Input: part model. Units: mm. Frame: model coordinates. A direction names the side the tool comes from. Coordinates: 2 decimals unless noted, no trailing zeros. Order: outer loops, then holes, each group sorted by start corner. A loop starts at its lowest first (then second) coordinate and runs counter-clockwise, first axis right, second up. Notation, with made-up numbers: (88.5, 41.25) -> (120.5, 41.25) arc R24 ccw to (120.5, 65.25) -> close; hole circle Ø1 at (-30, 18). An arc over 180 degrees is marked (long way). Use one line per item in the form item = value. Start each with the question number.
1) Draft query along Z for faces 4 (the cylindrical face through (16.6, 3.52, 19.93)), 5 (the cylindrical face through (0.96, 5.74, 9.23)), 6 (the cylindrical face through (-18.63, 0.6, 0.26)). Return one class per face: pulls with the +Z half, pulls with the -Z half, needs draft (parallel to the pull), parting line crosses it, or undercut.
2) Access query for faces 1 (the flat face through (0, 3, -15)), 2 (the cylindrical face through (0.96, 5.74, -16.77)), 3 (the flat face through (-17, 18, 0.5)). Directions: +Z, -Z, +X, -X, +Y, -Y. A direction counts if a zero-diameter tool reaches every point of the face in a straight line with its end or side. Return the directions, or none.
3) Section query D-D on z = 6. Output: boundary loops of the cut face in (x, y).
4) Section query B-B on z = 13. Output: boundary loops of the cut face in (x, y).
5) Section query A-A on y = 23.5. Output: boundary loops of the cut face in (x, z), then the cut area to 3 significant figures.
6) Pin query (flat end, axial travel): pin 1 (18 mm diameter, centred on x = -4, z = 3, fed in from +Y); pin 2 (12 mm diameter, centred on x = 9, y = 13, fed in from +Z); pin 3 (1 mm diameter, centred on x = 9, z = -6.5, fed in from +Y). Return the tip coordinate at first contact, or that it passes through.
7) Ray query, line 1 along X through (y, z) = (6.2, 13); line 2 along Z through (x, y) = (-1, 6.55); line 3 along X through (y, z) = (5.25, -13). Return the intervals inside material, ascending.
8) Section query C-C on x = -1. Count the separate pieces of the cut face and the enclosed holes in it, then the cut area to 3 significant figures.
Autodesk Inventor part; units mm, degrees
ref_plane "YZ Plane" through (0, 0, 0) normal (1, 0, 0) x (0, 1, 0)
ref_plane "XZ Plane" through (0, 0, 0) normal (0, 1, 0) x (-1, 0, 0)
ref_plane "XY Plane" through (0, 0, 0) normal (0, 0, 1) x (1, 0, 0)
sketch "Sketch1" plane through (0, 0, 0) normal (0, 1, 0) x (-1, 0, 0)
  line L0 (19.2, 20.5) -> (-17.2, 20.5)
  line L1 (-17.2, 20.5) -> (-17.2, -20.5)
  line L2 (-17.2, -20.5) -> (19.2, -20.5)
  line L3 (19.2, -20.5) -> (19.2, 20.5)
  point P0 (0, 0)
  dimension "d0" = 36.4
  dimension "d1" = 41
extrude "Extrusion1" add sketch "Sketch1" along normal blind 5
sketch "Sketch2" plane through (0, 5, 0) normal (0, 1, 0) x (1, 0, 0)
  line L0 (-19.2, -20.5) -> (17.2, -20.5)
  line L1 (-19.2, -20.5) -> (-14.2, -20.5)
  line L2 (-14.2, -20.5) -> (-14.2, -0.5)
  line L3 (-14.2, -0.5) -> (-19.2, -0.5)
  line L4 (-19.2, -0.5) -> (-19.2, -20.5)
  line L5 (17.2, 20.5) -> (-19.2, 20.5)
  line L6 (17.2, 20.5) -> (12.2, 20.5)
  line L7 (12.2, 20.5) -> (12.2, 0.5)
  line L8 (12.2, 0.5) -> (17.2, 0.5)
  line L9 (17.2, 0.5) -> (17.2, 20.5)
  point P0 (0, 0)
  dimension "d4" = 5
  dimension "d5" = 20
  dimension "d6" = 5
  dimension "d7" = 20
extrude "Extrusion2" add sketch "Sketch2" along normal blind 25.4
sketch "Sketch3" plane through (0, 5, 0) normal (0, 1, 0) x (1, 0, 0)
  circle A0 centre (-1, -13) radius 4.25
  circle A1 centre (-1, 13) radius 4.25
  line L0 (-14.2, -20.5) -> (-14.2, -0.5)
  line L1 (12.2, 20.5) -> (12.2, 0.5)
  point P0 (0, 0)
  dimension "d10" = 8.5
  dimension "d11" = 8.5
  dimension "d24" = 13.2
  dimension "d25" = 13.2
extrude "Extrusion3" add sketch "Sketch3" along normal blind 3
sketch "Sketch4" plane through (-1, 8, 13) normal (0, 1, 0) x (1, 0, 0)
  circle A0 centre (0, 0) radius 4.25
  circle A1 centre (0, 0) radius 2
  circle A2 centre (0, 26) radius 4.25
  circle A3 centre (0, 26) radius 2
  point P0 (1, 13)
  dimension "d14" = 4
  dimension "d15" = 4
extrude "Extrusion4" cut sketch "Sketch4" against normal blind 10 contours A1 | A3
fillet "Fillet1" radius 2 8 edges at (17.2, 0, 0) (-1, 0, 20.5) (-19.2, 0, 0) (-1, 0, -20.5) (-19.2, 15.2, 20.5) (17.2, 15.2, -20.5) (-19.2, 2.5, -20.5) (17.2, 2.5, 20.5)
fillet "Fillet2" radius 1.5 2 edges at (-5.25, 8, -13) (-5.25, 8, 13)
sketch "Sketch5" plane through (0, 0, 0) normal (0, -1, 0) x (1, 0, 0)
  circle A0 centre (-1, 13) radius 2
  circle A1 centre (-1, 13) radius 3
  circle A2 centre (-1, -13) radius 2
  circle A3 centre (-1, -13) radius 3
  point P0 (0, 0)
  dimension "d20" = 6
  dimension "d21" = 6
extrude "Extrusion5" cut sketch "Sketch5" against normal blind 3 contours A0 | A1 | A2 | A3
properties part number "botMountThick"
Answers below:
q1.face_4 = pulls with the +Z half
q1.face_5 = undercut
q1.face_6 = needs draft
q2.face_1 = -Y
q2.face_2 = +Y
q2.face_3 = -Z, +X, -X, +Y
q3.outline = (-19.2, 2) arc R2 ccw to (-17.2, 0) -> (15.2, 0) arc R2 ccw to (17.2, 2) -> (17.2, 5) -> (-14.2, 5) -> (-14.2, 30.4) -> (-19.2, 30.4) -> close
q4.outline = (-19.2, 2) arc R2 ccw to (-17.2, 0) -> (-4, 0) -> (-4, 3) -> (-3, 3) -> (-3, 8) -> (-3.75, 8) arc R1.5 ccw to (-5.25, 6.5) -> (-5.25, 5) -> (-14.2, 5) -> (-14.2, 30.4) -> (-19.2, 30.4) -> close; (1, 3) -> (2, 3) -> (2, 0) -> (15.2, 0) arc R2 ccw to (17.2, 2) -> (17.2, 5) -> (3.25, 5) -> (3.25, 6.5) arc R1.5 ccw to (1.75, 8) -> (1, 8) -> close
q5.outline = (-19.2, 0.5) -> (-14.2, 0.5) -> (-14.2, 20.5) -> (-17.2, 20.5) arc R2 ccw to (-19.2, 18.5) -> close; (12.2, -20.5) -> (15.2, -20.5) arc R2 ccw to (17.2, -18.5) -> (17.2, -0.5) -> (12.2, -0.5) -> close
q5.area = 198 mm^2
q6.pin_1 = 8
q6.pin_2 = -0.5
q6.pin_3 = 5
q7.line_1 = -19.2 to -14.2, -5.25 to -3, 1 to 3.25
q7.line_2 = -17.25 to -15, -11 to -8.75, 8.75 to 11, 15 to 17.25
q7.line_3 = -5.25 to -3, 1 to 3.25, 12.2 to 17.2
q8.separate_pieces = 3
q8.enclosed_holes = 0
q8.area = 176 mm^2
